from build123d import *

# Parameters (mm, degrees)
BOSS_EXTRUDE1_DEPTH = 10.16
CUT_EXTRUDE1_DEPTH  = 11.16
SKETCH4_W           = 129.547530324
SKETCH4_H           = 444.037072
CUT_EXTRUDE3_DEPTH  = 11.16
SKETCH5_W           = 10.16
SKETCH5_H           = 84.922739191
CUT_EXTRUDE5_DEPTH  = 11.16
CUT_EXTRUDE6_DEPTH  = 11.16
SKETCH11_R          = 3.175
SKETCH11_W          = 25.4
SKETCH11_H          = 50.8
CUT_EXTRUDE8_DEPTH  = 11.16


with BuildPart() as part:
    # Sketch1 → Boss-Extrude1 (new body)
    with BuildSketch(Plane.XY):
        with BuildLine():
            Line((20.32, 73.849956434), (0, 73.849956434))
            Line((0, 73.849956434), (0, 10.164894956))
            Line((0, 10.164894956), (20.32, 10.164894956))
            Line((20.32, 10.164894956), (115.06781826, 14.091181531))
            Line((115.06781826, 14.091181531), (115.488322648, 3.943711998))
            Line((115.488322648, 3.943711998), (210.656645296, 7.887423995))
            Line((210.656645296, 7.887423995), (210.236140908, 18.034893528))
            Line((210.236140908, 18.034893528), (305.404463556, 21.978605526))
            Line((305.404463556, 21.978605526), (305.824967945, 11.831135993))
            Line((305.824967945, 11.831135993), (400.993290593, 15.77484799))
            Line((400.993290593, 15.77484799), (400.572786204, 25.922317523))
            Line((400.572786204, 25.922317523), (495.741108852, 29.866029521))
            Line((495.741108852, 29.866029521), (496.161613241, 19.718559988))
            Line((496.161613241, 19.718559988), (591.329935889, 23.662271985))
            Line((591.329935889, 23.662271985), (590.909431501, 33.809741518))
            Line((590.909431501, 33.809741518), (686.077754149, 37.753453516))
            Line((686.077754149, 37.753453516), (686.498258538, 27.605983983))
            Line((686.498258538, 27.605983983), (781.666581186, 31.54969598))
            Line((781.666581186, 31.54969598), (781.246076797, 41.697165514))
            Line((781.246076797, 41.697165514), (781.246076797, 471.95159927))
            ThreePointArc((781.246076797, 471.95159927), (401.049995582, 500.057636465), (20.32, 519.645386783))
            Line((20.32, 519.645386783), (20.32, 455.960325305))
            Line((20.32, 455.960325305), (0, 455.960325305))
            Line((0, 455.960325305), (0, 392.275263826))
            Line((0, 392.275263826), (20.32, 392.275263826))
            Line((20.32, 392.275263826), (20.32, 328.590202348))
            Line((20.32, 328.590202348), (0, 328.590202348))
            Line((0, 328.590202348), (0, 264.905140869))
            Line((0, 264.905140869), (20.32, 264.905140869))
            Line((20.32, 264.905140869), (20.32, 201.220079391))
            Line((20.32, 201.220079391), (0, 201.220079391))
            Line((0, 201.220079391), (0, 137.535017912))
            Line((0, 137.535017912), (20.32, 137.535017912))
            Line((20.32, 137.535017912), (20.32, 73.849956434))
        make_face()
    extrude(amount=BOSS_EXTRUDE1_DEPTH)

    # Sketch2 → Cut-Extrude1 (cut, through all)
    with BuildSketch(Plane.XY.offset(10.16)):
        Polygon((20.32, 471.23904919), (781.246076797, 460.948390721), (781.246076797, 535.017906983), (20.32, 535.017906983), align=None)
    extrude(amount=-CUT_EXTRUDE1_DEPTH, mode=Mode.SUBTRACT)

    # Sketch4 → Cut-Extrude3 (cut, through all)
    with BuildSketch(Plane(origin=(0, 0, 0), x_dir=(-1, 0, 0), z_dir=(0, 0, -1))):
        with Locations((-751.2720237, 249.624519983)):
            Rectangle(SKETCH4_W, SKETCH4_H)
    extrude(amount=-CUT_EXTRUDE3_DEPTH, mode=Mode.SUBTRACT)

    # Sketch5 → Cut-Extrude5 (cut, through all)
    with BuildSketch(Plane(origin=(0, 0, 0), x_dir=(-1, 0, 0), z_dir=(0, 0, -1))):
        Polygon((-686.498258538, 122.676192707), (-686.498258538, 37.753453516), (-686.077754149, 37.753453516), (-676.338258538, 37.753453516), (-676.338258538, 122.676192707), align=None)
        with Locations((-681.418258538, 250.060301493)):
            Rectangle(SKETCH5_W, SKETCH5_H)
        Polygon((-686.498258538, 462.229747042), (-686.498258538, 377.444410279), (-676.338258538, 377.444410279), (-676.338258538, 462.367149469), align=None)
        Polygon((-676.338258538, 37.349855295), (-686.077754149, 37.753453516), (-686.498258538, 27.605983983), (-686.498258538, 26.157835014), (-676.338258538, 26.157835014), align=None)
        Polygon((-686.077754149, 37.753453516), (-686.498258538, 37.753453516), (-686.498258538, 27.605983983), align=None)
        Polygon((-676.338258538, 37.753453516), (-686.077754149, 37.753453516), (-676.338258538, 37.349855295), align=None)
    extrude(amount=-CUT_EXTRUDE5_DEPTH, mode=Mode.SUBTRACT)

    # Sketch9 → Cut-Extrude6 (cut, through all)
    with BuildSketch(Plane(origin=(0, 0, 0), x_dir=(-1, 0, 0), z_dir=(0, 0, -1))):
        Polygon((-248.83741583, 457.991507139), (-248.974805694, 468.150578161), (-325.167838357, 467.12015418), (-325.030448493, 456.961083159), align=None)
        Polygon((-96.52, 470.208530984), (-96.52, 460.048530984), (-172.713032663, 459.018107004), (-172.713032663, 469.178107004), align=None)
    extrude(amount=-CUT_EXTRUDE6_DEPTH, mode=Mode.SUBTRACT)

    # Sketch11 → Cut-Extrude8 (cut, through all)
    with BuildSketch(Plane.XY.offset(10.16)):
        with Locations((366.619369126, 431.770831078)):
            Circle(SKETCH11_R)
        with Locations((366.619369126, 380.970831078)):
            Circle(SKETCH11_R)
        with Locations((239.619369126, 431.770831078)):
            Circle(SKETCH11_R)
        with Locations((239.619369126, 380.970831078)):
            Circle(SKETCH11_R)
        with Locations((265.019369126, 406.370831078)):
            Circle(SKETCH11_R)
        with Locations((341.219369126, 406.370831078)):
            Circle(SKETCH11_R)
        with Locations((265.019369126, 355.570831078)):
            Circle(SKETCH11_R)
        with Locations((341.219369126, 355.570831078)):
            Circle(SKETCH11_R)
        with Locations((303.119369126, 406.370831078)):
            Rectangle(SKETCH11_W, SKETCH11_H)
    extrude(amount=-CUT_EXTRUDE8_DEPTH, mode=Mode.SUBTRACT)


solid = part.part
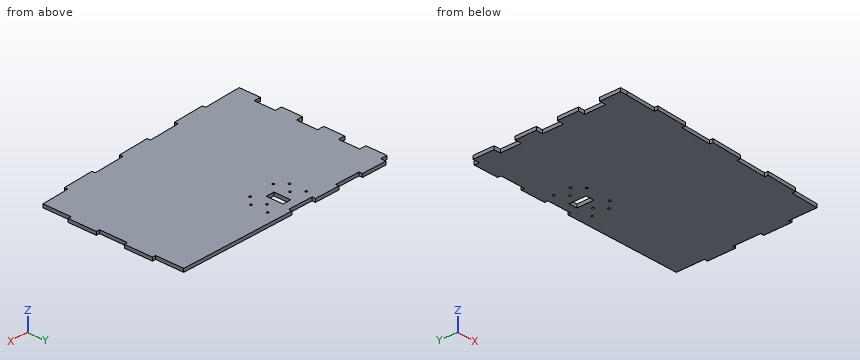
Geometry check sheet. Reference: the model listing, model coordinates, mm. Round coordinates to 2 decimals unless told otherwise and drop trailing zeros. Order: outer loops, then holes, each group sorted by start corner. A loop starts at its lowest first (then second) coordinate and runs counter-clockwise, first axis right, second up. Notation, with made-up numbers: M 0.5,-14 L 15.5,-14 A10 cw 15.5,0 Z; hole C 72.5,53.5 d10. An arc over 180 degrees is marked long. Answer in a Markdown table with one row per item. Add a question column.
Item 1: Sectioned sample at C-C, the plane z = 6. State how many separate pieces and enclosed holes the cut face has, plus the area to 3 significant figures.
Item 2: Sectioned sample at A-A, the plane y = 341. Enter the section's corners in (x, z).
Item 3: Material ranges on L1, parallel to X at y = 412.5, z = 2.5; L2, parallel to X at y = 102, z = 7.25; L3, parallel to X at y = 49, z = 6.75, recorded low to high. Write a range as [from, to].
Item 4: Depth check by flat-ended pin: pin 1 Ø5 at (y, z) = (424.5, 6.5) entering from +X; pin 2 Ø2 at (y, z) = (132, 4) entering from -X; pin 3 Ø5 at (x, z) = (10, 3.5) entering from -Y. Enter the tip coordinate at first touch or a pass-through.
Item 5: Sectioned sample at B-B, the plane x = 52. Enter the section's corners in (y, z), plus the area to 3 significant figures.
Filled in:
| question | item | result |
|---|---|---|
| 1 | separate pieces | 1 |
| 1 | enclosed holes | 9 |
| 1 | area | 297,000 mm² |
| 2 | outline | M 20.32,0 L 686.5,0 L 686.5,10.16 L 20.32,10.16 Z |
| 3 | L1 | x = [0, 290.42], [315.82, 676.34] |
| 3 | L2 | x = [20.32, 676.34] |
| 3 | L3 | x = [0, 676.34] |
| 4 | pin 1 | stops at x = 676.34 |
| 4 | pin 2 | stops at x = 20.32 |
| 4 | pin 3 | stops at y = 10.16 |
| 5 | outline | M 11.48,0 L 470.81,0 L 470.81,10.16 L 11.48,10.16 Z |
| 5 | area | 4,670 mm² |
